Geometry: final body of the model. Coordinates: model frame, mm. A direction names the side the tool comes from. Coordinates: 2 decimals unless noted, no trailing zeros. Order: outer loops, then holes, each group sorted by start corner. A loop starts at its lowest first (then second) coordinate and runs counter-clockwise, first axis right, second up. Notation, with made-up numbers: (-20.5, 50) -> (36.5, 50) arc R21 cw to (36.5, 80) -> close; hole circle Ø9 at (-27, 87.25). An arc over 180 degrees is marked (long way). Answer in a Markdown table with one row per item. Add a question column.
1) Pull-direction query (X, two-part tool) for faces 1 (the face through (8, -2, -1)), 2 (the face through (-2, 8, -1)), 3 (the face through (0, 1, -1)), 4 (the face through (-8, 0, -8)); classes: +X half, -X half, draft (parallel to the pull), parting line (faces both ways), or undercut.
2) Section query C-C on y = 11. Return the cut outline in (x, z).
3) Set-up query: faces 5 (the face through (8, 2, -1)), 6 (the face through (0.084, 0.014, -2.043)), 7 (the face through (-10, 2, -2)), 8 (the face through (10, 2, -2)), 9 (the face through (2, 12, -2)). Return all of +Z, -Z, +X, -X, +Y, -Y with unobstructed straight access to the full face (end or side cutting, diameter ignored); none if empty.
4) Ray query, line 1 (Y direction, x = 0, z = -0.55); line 2 (Y direction, x = 11, z = -1.3); line 3 (Z direction, x = 8.75, y = 0.75). Return the intervals inside material, ascending. Write a range as from..to.
5) Contact query for flat-ended pins moving along their axis: P1, Ø6, axis at x = 5.5, z = -9.5, coming from the +Y side; P2, Ø1, axis at x = 2, z = -0.5, coming from the -Y side; P3, Ø7.5, axis at y = 5, z = -5.5, coming from the -X side. Output: stop coordinate, or through.
6) Section query B-B on x = -4.75. Return the cut outline in (y, z).
7) Section query D-D on x = 0. Return the cut outline in (y, z).
8) Section query A-A on z = -4.5. Return the cut outline in (x, y), then the cut area to 3 significant figures.
```python
from build123d import *

# Parameters (mm, degrees)
SKETCH6_W           = 12
SKETCH6_H           = 8
BOSS_EXTRUDE5_DEPTH = 1
SKETCH7_W           = 6
SKETCH7_H           = 2
BOSS_EXTRUDE6_DEPTH = 2
SKETCH8_W           = 12
SKETCH8_H           = 10
CUT_EXTRUDE4_DEPTH  = 2.5
BOSS_EXTRUDE7_DEPTH = 1
SKETCH12_W          = 6
SKETCH12_H          = 6
BOSS_EXTRUDE9_DEPTH = 2
SKETCH13_R          = 2
CUT_EXTRUDE7_DEPTH  = 25.248711306


with BuildPart() as part:
    # Sketch6 → Boss-Extrude5 (new, symmetric)
    with BuildSketch(Plane(origin=(0, 0, 0), x_dir=(1, 0, 0), z_dir=(0, 1, 0))):
        Polygon((-14, 0), (14, 0), (14, 2), (8, 2), (8, 14), (-8, 14), (-8, 2), (-14, 2), align=None)
        with Locations((0, 8)):
            Rectangle(SKETCH6_W, SKETCH6_H, mode=Mode.SUBTRACT)
    extrude(amount=BOSS_EXTRUDE5_DEPTH, both=True)

    # Sketch7 → Boss-Extrude6 (add)
    with BuildSketch(Plane(origin=(0, 0, -2), x_dir=(-1, 0, 0), z_dir=(0, 0, -1))):
        with Locations((11, 2)):
            Rectangle(SKETCH7_W, SKETCH7_H)
        with Locations((11, -2)):
            Rectangle(SKETCH7_W, SKETCH7_H)
    boss_extrude6 = extrude(amount=-BOSS_EXTRUDE6_DEPTH)

    # Mirror2: Boss-Extrude6 across plane
    add(boss_extrude6.mirror(Plane(origin=(0, 0, 0), x_dir=(0, 0, 1), z_dir=(1, 0, 0))))

    # Sketch8 → Cut-Extrude4 (cut, symmetric)
    with BuildSketch(Plane(origin=(0, -0.265057015, 0.016211582), x_dir=(-1, 0, 0), z_dir=(0, 0.9981347984218666, -0.061048539534864034))):
        with Locations((0, -7.038666121)):
            Rectangle(SKETCH8_W, SKETCH8_H)
    extrude(amount=CUT_EXTRUDE4_DEPTH, both=True, mode=Mode.SUBTRACT)

    # Sketch10 → Boss-Extrude7 (add, symmetric)
    with BuildSketch(Plane(origin=(0, 0, 0), x_dir=(0, 0, -1), z_dir=(1, 0, 0))):
        Polygon((12.12232524, 1), (12.428138341, 6), (0, 6), (0, 14), (2, 14), (2, 8), (14, 8), (14, 1), align=None)
    extrude(amount=BOSS_EXTRUDE7_DEPTH, both=True)

    # Sketch12 → Boss-Extrude9 (add)
    with BuildSketch(Plane(origin=(0, 0, -2), x_dir=(-1, 0, 0), z_dir=(0, 0, -1))):
        with Locations((0, 11)):
            Rectangle(SKETCH12_W, SKETCH12_H)
    extrude(amount=-BOSS_EXTRUDE9_DEPTH)

    # Sketch13 → Cut-Extrude7 (cut, through all)
    with BuildSketch(Plane.XY):
        with Locations((-11, 0)):
            Circle(SKETCH13_R)
        with Locations((11, 0)):
            Circle(SKETCH13_R)
        with Locations((0, 11)):
            Circle(SKETCH13_R)
    extrude(amount=-CUT_EXTRUDE7_DEPTH, mode=Mode.SUBTRACT)


solid = part.part
```
Result:
| question | item | result |
|---|---|---|
| 1 | face 1 | undercut |
| 1 | face 2 | draft |
| 1 | face 3 | undercut |
| 1 | face 4 | -X half |
| 2 | outline | (-3, -2) -> (-2, -2) -> (-2, 0) -> (-3, 0) -> close; (2, -2) -> (3, -2) -> (3, 0) -> (2, 0) -> close |
| 3 | face 5 | +Z, -Z, +Y |
| 3 | face 6 | -Y |
| 3 | face 7 | -Z, -X, +Y, -Y |
| 3 | face 8 | -Z, +X, +Y, -Y |
| 3 | face 9 | -Z, +X, -X, +Y |
| 4 | line 1 | -1..1, 6..9, 13..14 |
| 4 | line 2 | -3..-2, 2..3 |
| 4 | line 3 | -2..0 |
| 5 | P1 | y = 1 |
| 5 | P2 | y = -1 |
| 5 | P3 | x = -1 |
| 6 | outline | (-1, -14) -> (1, -14) -> (1, -12.12) -> (-1, -12) -> close; (-1, -1.98) -> (1, -2.1) -> (1, 0) -> (-1, 0) -> close |
| 7 | outline | (-1, -14) -> (8, -14) -> (8, -2) -> (9, -2) -> (9, 0) -> (6, 0) -> (6, -12.43) -> (-1, -12) -> close; (-1, -1.98) -> (1, -2.1) -> (1, 0) -> (-1, 0) -> close; (13, -2) -> (14, -2) -> (14, 0) -> (13, 0) -> close |
| 8 | outline | (-8, -1) -> (-6, -1) -> (-6, 1) -> (-8, 1) -> close; (-1, 6) -> (1, 6) -> (1, 8) -> (-1, 8) -> close; (6, -1) -> (8, -1) -> (8, 1) -> (6, 1) -> close |
| 8 | area | 12.0 mm2 |
